```python
from build123d import *

# Parameters (mm, degrees)
EXTRUDE_1_DEPTH     = 5.5
SKETCH_2_R          = 1.55
CUT_EXTRUDE_1_DEPTH = 65.217448119


with BuildPart() as part:
    # ｽｹｯﾁ1 → ﾎﾞｽ - 押し出し1 (new body)
    with BuildSketch(Plane.XY):
        with BuildLine():
            Line((-60, 5), (-47.033321686, 5))
            Line((-47.033321686, 5), (-33.07098347, -11))
            Line((-33.07098347, -11), (-28.618176043, -11))
            ThreePointArc((-28.618176043, -11), (0, 10), (28.618176043, -11))
            Line((28.618176043, -11), (33.07098347, -11))
            Line((33.07098347, -11), (47.033321686, 5))
            Line((47.033321686, 5), (60, 5))
            Line((60, 5), (60, -5))
            Line((60, -5), (44.942957201, -5))
            Line((44.942957201, -5), (29.917910397, -22.217800138))
            Line((29.917910397, -22.217800138), (19.876653706, -22.217800138))
            ThreePointArc((19.876653706, -22.217800138), (0, 0), (-19.876653706, -22.217800138))
            Line((-19.876653706, -22.217800138), (-29.917910397, -22.217800138))
            Line((-29.917910397, -22.217800138), (-44.942957201, -5))
            Line((-44.942957201, -5), (-60, -5))
            Line((-60, -5), (-60, 5))
        make_face()
    extrude(amount=EXTRUDE_1_DEPTH)

    # ｽｹｯﾁ2 → ｶｯﾄ - 押し出し1 (cut, through all)
    with BuildSketch(Plane.XY.offset(5.5)):
        with Locations((-55, 0)):
            Circle(SKETCH_2_R)
        with Locations((55, 0)):
            Circle(SKETCH_2_R)
    extrude(amount=-CUT_EXTRUDE_1_DEPTH, mode=Mode.SUBTRACT)


solid = part.part
```
The listing builds one solid part. Answer for the finished solid, in the listing's coordinates (mm). A direction names the side the tool comes from. Give positions to 0.01 mm unless a question says otherwise; leave off trailing zeros. Order: outer loops, then holes, each group sorted by start corner. A loop starts at its lowest first (then second) coordinate and runs counter-clockwise, first axis right, second up. Notation, with made-up numbers: (-21.5, -38) -> (24.5, -38) arc R28 ccw to (24.5, -1) -> close; hole circle Ø2 at (73, 65.5). An arc over 180 degrees is marked (long way). One line per item, written item: value.
1) Find section A-A, the plane x = 55. Determine the outline of the cut face in (y, z).
Reported:
outline: (-5, 0) -> (-1.55, 0) -> (-1.55, 5.5) -> (-5, 5.5) -> close; (1.55, 0) -> (5, 0) -> (5, 5.5) -> (1.55, 5.5) -> close
2) Find section C-C, the plane y = -9.5. Determine the outline of the cut face in (x, z).
Reported:
outline: (-41.02, 0) -> (-34.38, 0) -> (-34.38, 5.5) -> (-41.02, 5.5) -> close; (-28.1, 0) -> (-17.02, 0) -> (-17.02, 5.5) -> (-28.1, 5.5) -> close; (17.02, 0) -> (28.1, 0) -> (28.1, 5.5) -> (17.02, 5.5) -> close; (34.38, 0) -> (41.02, 0) -> (41.02, 5.5) -> (34.38, 5.5) -> close
3) Find section D-D, the plane y = -20. Determine the outline of the cut face in (x, z).
Reported:
outline: (-31.85, 0) -> (-20, 0) -> (-20, 5.5) -> (-31.85, 5.5) -> close; (20, 0) -> (31.85, 0) -> (31.85, 5.5) -> (20, 5.5) -> close
4) A tool of negligible diameter and unlimited length cuts with its end or side. For faces 1 (the flat face through (39.954, -3.112, 2.712)), 2 (the flat face through (53, -5, 3)), 3 (the cylindrical face through (56.478, 0.466, 2.788)), 4 (the flat face through (-54, 5, 3)), 5 (the flat face through (53, 5, 3)), from which of +Z, -Z, +X, -X, +Y, -Y can it reach the whole face along a straight path? Write none if from no direction.
Reported:
face 1: +Z, -Z, +Y
face 2: +Z, -Z, +X, -Y
face 3: +Z, -Z
face 4: +Z, -Z, -X, +Y
face 5: +Z, -Z, +X, +Y
5) Flat-ended cylindrical pins translate along their axes: P1, Ø10, axis at x = -29.5, y = -10.5, coming from the +Z side; P2, Ø2, axis at x = -31, z = 3.5, coming from the +Y side; P3, Ø1.6, axis at x = 53.5, z = 3, coming from the +Y side. Find the tip coordinate at first contact, or state that the pin passes through.
Reported:
P1: stops at z = 5.5
P2: stops at y = -11
P3: stops at y = 5
6) Find section B-B, the plane z = 1.9. Determine the outline of the cut face in (x, y).
Reported:
outline: (-60, -5) -> (-44.94, -5) -> (-29.92, -22.22) -> (-19.88, -22.22) arc R20 cw (long way) to (19.88, -22.22) -> (29.92, -22.22) -> (44.94, -5) -> (60, -5) -> (60, 5) -> (47.03, 5) -> (33.07, -11) -> (28.62, -11) arc R30 ccw to (-28.62, -11) -> (-33.07, -11) -> (-47.03, 5) -> (-60, 5) -> close; hole circle Ø3.1 at (-55, 0); hole circle Ø3.1 at (55, 0)
7) Determine the mould class of faces 6 (the cylindrical face through (-53.522, 0.466, 2.788)), 7 (the cylindrical face through (-0.532, 9.995, 2.712)), 8 (the flat face through (-52, -5, 3)) for opening direction Y: pulls with the +Y half, pulls with the -Y half, needs draft (parallel to the pull), parting line crosses it, or undercut.
Reported:
face 6: undercut
face 7: pulls with the +Y half
face 8: pulls with the -Y half
8) Find the intervals of material crossed by line 1 (X direction, y = 4.5, z = 4.85); line 2 (X direction, y = -7, z = 2.65); line 3 (X direction, y = -2.5, z = 4.5), in increasing order.
Reported:
line 1: x = -60 to -46.6, -17.31 to 17.31, 46.6 to 60
line 2: x = -43.2 to -36.56, -27.04 to -15.2, 15.2 to 27.04, 36.56 to 43.2
line 3: x = -60 to -40.49, -24.37 to -9.68, 9.68 to 24.37, 40.49 to 60
